Input: dimensioned drawing with shaded views. Units: mm. Origin: part minimum x, y, z. A direction names the side the tool comes from. Coordinates: 2 decimals unless noted, no trailing zeros. Order: outer loops, then holes, each group sorted by start corner. A loop starts at its lowest first (then second) coordinate and runs counter-clockwise, first axis right, second up. Notation, with made-up numbers: M 74,76.5 L 88,76.5 A17 cw 88,92.5 Z; hole C 26.5,-19 d7. An arc over 180 degrees is marked long. Write item = value, one per line.
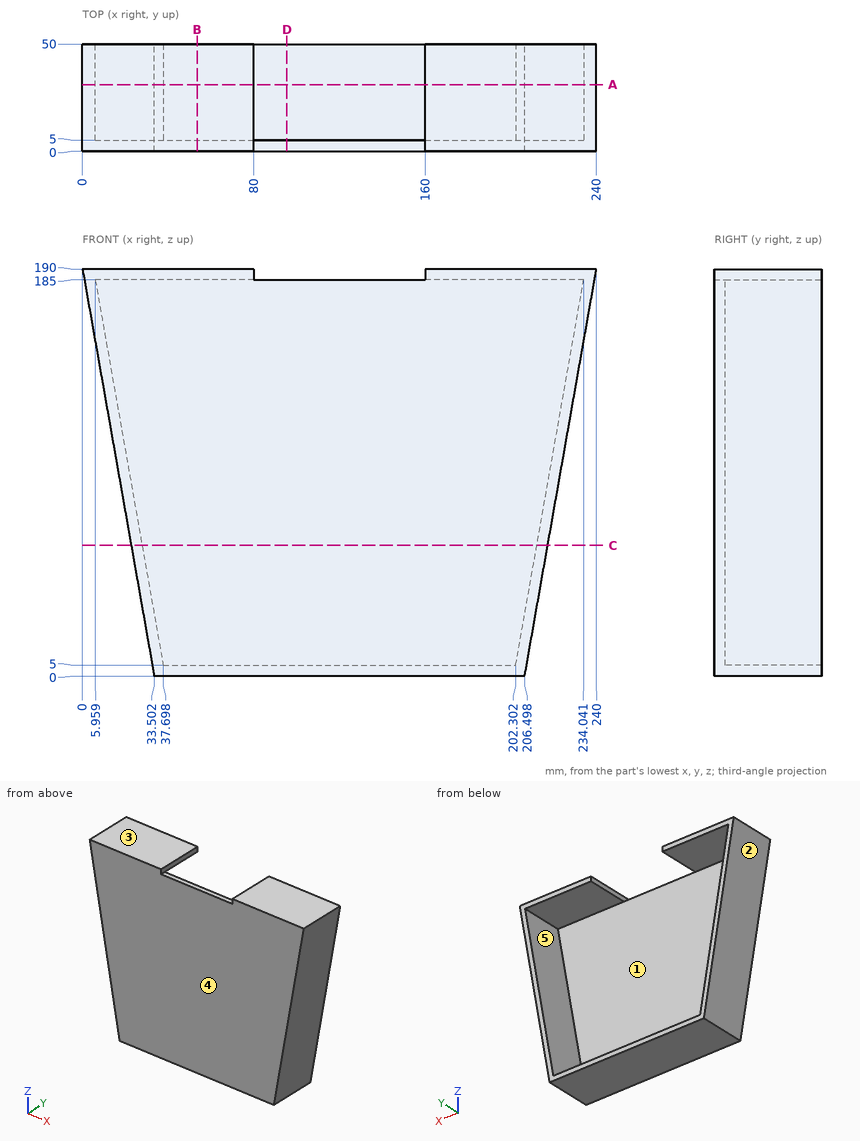
1) Section B-B, the plane x = 53.5. Return loops of the section in (y, z), and give its area (3 significant figures).
Numbers:
outline = M 0,0 L 50,0 L 50,5 L 5,5 L 5,185 L 50,185 L 50,190 L 0,190 Z
area = 1,400 mm²
2) Section D-D, the plane x = 95.5. Return loops of the section in (y, z).
Numbers:
outline = M 0,0 L 50,0 L 50,5 L 5,5 L 5,185 L 0,185 Z
3) Line query: L1, parallel to Z at x = 43, y = 38.5; L2, parallel to Y at x = 165, z = 110; L3, parallel to X at y = 29, z = 60. Output: solid intervals per line, ascending.
Numbers:
L1 = 0 to 5, 185 to 190
L2 = 0 to 5
L3 = 22.92 to 28, 212 to 217.08
4) Pin query (flat end, axial travel): pin 1 (2.5 mm diameter, centred on y = 26.5, z = 186.5, fed in from -X); pin 2 (1.5 mm diameter, centred on x = 103.5, y = 30.5, fed in from +Z); pin 3 (5 mm diameter, centred on y = 41, z = 79, fed in from -X); pin 4 (5 mm diameter, centred on x = 212, z = 68.5, fed in from -Y). Return the tip coordinate at first contact, or that it passes through.
Numbers:
pin_1 = 0.4
pin_2 = 5
pin_3 = 19.13
pin_4 = 0
5) Mould query, pull axis Z, two halves, no side actions, for the marked faces 1, 2 and 3. Classes: pulls with the +Z half, pulls with the -Z half, needs draft (parallel to the pull), parting line crosses it, or undercut.
Numbers:
face_1 = undercut
face_2 = pulls with the -Z half
face_3 = pulls with the +Z half
6) Section C-C, the plane z = 61. Return loops of the section in (x, y).
Numbers:
outline = M 22.75,0 L 217.25,0 L 217.25,50 L 212.18,50 L 212.18,5 L 27.82,5 L 27.82,50 L 22.75,50 Z
7) Set-up query: the marked faces 4 and 5. Return all of +Z, -Z, +X, -X, +Y, -Y with unobstructed straight access to the full face (end or side cutting, diameter ignored); none if empty.
Numbers:
face_4 = +Z, -Z, +X, -X, -Y
face_5 = +Y
8) Section A-A, the plane y = 31. Return loops of the section in (x, z), and give its area (3 significant figures).
Numbers:
outline = M 0,190 L 33.5,0 L 206.5,0 L 240,190 L 160,190 L 160,185 L 234.04,185 L 202.3,5 L 37.7,5 L 5.96,185 L 80,185 L 80,190 Z
area = 3,490 mm²
